The listing builds one solid part. Answer for the finished solid, in the listing's coordinates (mm). Give positions to 0.01 mm unless a question says otherwise; leave off trailing zeros. Order: outer loops, then holes, each group sorted by start corner. A loop starts at its lowest first (then second) coordinate and runs counter-clockwise, first axis right, second up. Notation, with made-up numbers: (59, -24) -> (63, -24) arc R27 ccw to (63, 4) -> close; hole circle Ø1 at (11.5, 27). An arc over 180 degrees is marked (long way). Write item = value, one per line. Start each with the question number.
```python
from build123d import *

# Parameters (mm, degrees)
SKIZZE1_W                       = 25
SKIZZE1_H                       = 12
AUFSATZ_LINEAR_AUSTRAGEN1_DEPTH = 50
VERRUNDUNG1_R                   = 3


with BuildPart() as part:
    # Skizze1 → Aufsatz-Linear austragen1 (new body)
    with BuildSketch(Plane(origin=(0, 0, 0), x_dir=(1, 0, 0), z_dir=(0, 1, 0))):
        with Locations((12.5, 6)):
            Rectangle(SKIZZE1_W, SKIZZE1_H)
    extrude(amount=AUFSATZ_LINEAR_AUSTRAGEN1_DEPTH)

    # Verrundung1
    verrundung1_edges = [part.edges().sort_by_distance(p)[0] for p in [
        (0, 25, -12),
        (25, 25, -12),
        (25, 25, 0),
        (0, 25, 0),
    ]]
    fillet(verrundung1_edges, radius=VERRUNDUNG1_R)


solid = part.part
```
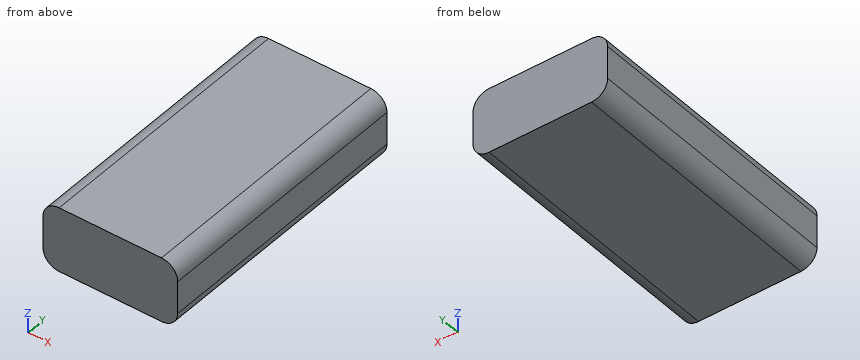
Item 1: A cutting plane is placed at A-A, the plane y = 7. Write down the section's boundary in (x, z).
Item 2: A cutting plane is placed at B-B, the plane z = -10.25. Write down the section's boundary in (x, y).
Item 3: Consider L1, parallel to X at y = 17, z = -9.25; L2, parallel to Z at x = 2.25, y = 4.5; L3, parallel to X at y = 19.5, z = -1.75. Determine where each line is inside the solid, lowest interval first. Write a range as from..to.
Item 4: A cutting plane is placed at C-C, the plane z = -0.75. Write down the section's boundary in (x, y).
Check values:
q1.outline = (0, -9) arc R3 ccw to (3, -12) -> (22, -12) arc R3 ccw to (25, -9) -> (25, -3) arc R3 ccw to (22, 0) -> (3, 0) arc R3 ccw to (0, -3) -> close
q2.outline = (0.27, 0) -> (24.73, 0) -> (24.73, 50) -> (0.27, 50) -> close
q3.L1 = 0.01..24.99
q3.L2 = -11.9..-0.1
q3.L3 = 0.27..24.73
q4.outline = (1.02, 0) -> (23.98, 0) -> (23.98, 50) -> (1.02, 50) -> close
